Model file for the job. Use its own axes, mm. Coordinates: 2 decimals unless noted, no trailing zeros. Write each loop counter-clockwise with the first axis right and the second up, starting at its lowest first coordinate (ties: lowest second). Pieces come first, ordered by that corner, then holes. Notation, with made-up numbers: M 64,-26 L 78,-26 A20 ccw 78,2 Z; hole C 30,-7.75 d9. An arc over 180 degrees is marked long. One line per question, with ' | ' between items. Start each with the question number.
(1) Cut at A-A (x = 42.5). Write the cut outline in (y, z).
(2) Cut at D-D (y = 15). Write the cut outline in (x, z), plus the area to 3 significant figures.
(3) Cut at C-C (z = 33). Write the cut outline in (x, y).
(4) Cut at B-B (z = 174). Write the cut outline in (x, y).
(5) Flat gauge pins, fed straight in: pin 1 Ø5 at (x, y) = (59, 3.5) entering from +Z; pin 2 Ø12 at (y, z) = (17, 116) entering from -X; pin 3 Ø3 at (x, y) = (58, 28) entering from -Z. Where does each tip first touch, or does it go through?
(6) Wall check: probe 1 along X at (y, z) = (4, 74.5); probe 2 along X at (y, z) = (8, 4); probe 3 along Z at (x, y) = (80.5, 8.5). Give the ranges that are in metal, low to high.
from build123d import *

# Parameters (mm, degrees)
SKETCH_1_W          = 99
SKETCH_1_H          = 79
SKETCH_1_R          = 2.5
SKETCH_1_W_2        = 81
SKETCH_1_H_2        = 61
EXTRUDE_1_DEPTH     = 10
EXTRUDE_2_DEPTH     = 15
CUT_EXTRUDE_1_DEPTH = 6
EXTRUDE_3_REACH     = 202.547
SKETCH_7_W          = 10
SKETCH_7_H          = 10
SKETCH_8_R          = 2.5
CUT_EXTRUDE_2_DEPTH = 206.898640112
FILLET_1_R          = 3


with BuildPart() as part:
    # 草图1 → 凸台-拉伸1 (new body)
    with BuildSketch(Plane(origin=(0, 0, 0), x_dir=(1, 0, 0), z_dir=(0, 1, 0))):
        with Locations((49.5, -39.5)):
            Rectangle(SKETCH_1_W, SKETCH_1_H)
        with Locations(Location((94.5, -4.5, 0), (0, 0, 270))):
            Circle(SKETCH_1_R, mode=Mode.SUBTRACT)
        with Locations(Location((4.5, -4.5, 0), (0, 0, 270))):
            Circle(SKETCH_1_R, mode=Mode.SUBTRACT)
        with Locations(Location((4.5, -74.5, 0), (0, 0, 270))):
            Circle(SKETCH_1_R, mode=Mode.SUBTRACT)
        with Locations(Location((94.5, -74.5, 0), (0, 0, 270))):
            Circle(SKETCH_1_R, mode=Mode.SUBTRACT)
        with Locations((49.5, -39.5)):
            Rectangle(SKETCH_1_W_2, SKETCH_1_H_2, mode=Mode.SUBTRACT)
    extrude(amount=EXTRUDE_1_DEPTH)

    # 草图4 → 凸台-拉伸2 (add)
    with BuildSketch(Plane(origin=(99, 0, 0), x_dir=(0, 0, -1), z_dir=(1, 0, 0))):
        Polygon((-79, 0), (-149, 23.5), (-179, 23.5), (-179, 33.5), (-149, 33.5), (-79, 10), align=None)
    extrude_2 = extrude(amount=-EXTRUDE_2_DEPTH)

    # 镜向1: 凸台-拉伸2 across plane
    add(extrude_2.mirror(Plane.ZY.offset(-49.5)))

    # 草图4<2> → 切除-拉伸1 (cut)
    with BuildSketch(Plane(origin=(99, 0, 0), x_dir=(0, 0, -1), z_dir=(1, 0, 0))):
        Polygon((-79, 0), (-149, 23.5), (-179, 23.5), (-179, 33.5), (-149, 33.5), (-79, 10), align=None)
    cut_extrude_1 = extrude(amount=-CUT_EXTRUDE_1_DEPTH, mode=Mode.SUBTRACT)

    # 镜向2: 切除-拉伸1 across plane
    add(cut_extrude_1.mirror(Plane.ZY.offset(-49.5)), mode=Mode.SUBTRACT)

    # 草图7 → 凸台-拉伸3 (add, up to next)
    with BuildSketch(Plane.ZY.offset(-84), mode=Mode.PRIVATE) as extrude_3_sk1:
        with Locations((174, 28.5)):
            Rectangle(SKETCH_7_W, SKETCH_7_H)
    extrude_3_tool1 = extrude(extrude_3_sk1.sketch, amount=EXTRUDE_3_REACH, mode=Mode.PRIVATE) - part.part
    add(extrude_3_tool1.solids().sort_by_distance((84, 28.5, 174))[0])

    # 草图8 → 切除-拉伸2 (cut, through all)
    with BuildSketch(Plane.XZ.offset(-23.5)):
        with Locations(Location((88, 174, 0), (0, 0, 270))):
            Circle(SKETCH_8_R)
        with Locations(Location((11, 174, 0), (0, 0, 270))):
            Circle(SKETCH_8_R)
    extrude(amount=-CUT_EXTRUDE_2_DEPTH, mode=Mode.SUBTRACT)

    # 圆角1
    fillet_1_edges = [part.edges().sort_by_distance(p)[0] for p in [
        (0, 5, 79),
        (6, 5, 79),
        (6, 28.5, 179),
        (0, 5, 0),
        (99, 5, 0),
        (93, 5, 79),
        (93, 28.5, 179),
        (99, 5, 79),
    ]]
    fillet(fillet_1_edges, radius=FILLET_1_R - 0.0001)  # a hair under: the kernel refuses the full size


solid = part.part
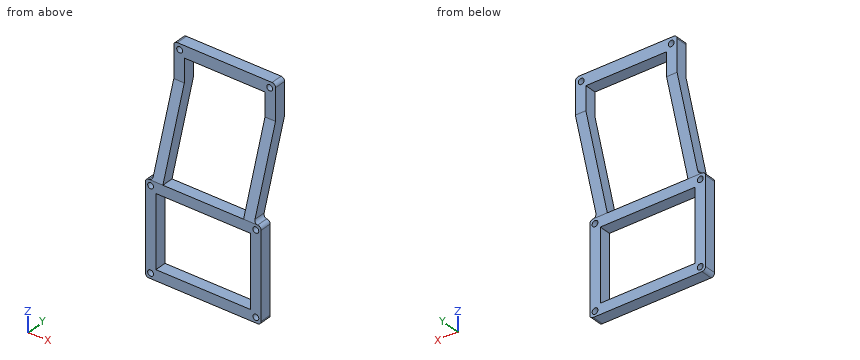
Filled in:
1) outline: M 0,0 L 10,0 L 10,9 L 0,9 Z; M 0,70 L 10,70 L 10,79 L 0,79 Z; M 23.5,169 L 33.5,169 L 33.5,179 L 23.5,179 Z
2) outline: M 6,93.89 L 15,93.89 L 15,123.68 L 6,123.68 Z; M 84,93.89 L 93,93.89 L 93,123.68 L 84,123.68 Z | area: 536 mm²
3) outline: M 0,0 L 9,0 L 9,10 L 0,10 Z; M 90,0 L 99,0 L 99,10 L 90,10 Z
4) outline: M 6,23.5 L 8.5,23.5 L 8.5,33.5 L 6,33.5 Z; M 13.5,23.5 L 85.5,23.5 L 85.5,33.5 L 13.5,33.5 Z; M 90.5,23.5 L 93,23.5 L 93,33.5 L 90.5,33.5 Z
5) pin 1: z = 79 | pin 2: x = 6 | pin 3: z = 169
6) probe 1: 0 to 2, 7 to 92, 97 to 99 | probe 2: 0 to 2.05, 6.95 to 92.05, 96.95 to 99 | probe 3: 0 to 9, 70 to 79
